Solid Edge part; units mm, degrees
sketch "Sketch1" plane through (0, 0, 0) normal (0, 0, 1) x (1, 0, 0)
  line L0 (0, 0) -> (50.8, 0)
  line L1 (50.8, 0) -> (50.8, 63.5)
  line L2 (50.8, 63.5) -> (0, 63.5)
  line L3 (0, 63.5) -> (0, 0)
extrude "Protrusion1" add sketch "Sketch1" along normal blind 3.175
hole "Hole_1" at (7.9375, 6.35, 0) direction (0, 0, 1) diameter 4.826 end up to next countersink diameter 9.525 countersink angle 82
hole "Hole1" at (42.8625, 6.35, 0) direction (0, 0, 1) diameter 4.826 end up to next countersink diameter 9.525 countersink angle 82
hole "Hole_2" at (25.4, 34.925, 3.175) direction (0, 0, -1) diameter 12.7 end up to next
chamfer "Chamfer_1" distance 6.35 angle 45 2 edges at (0, 63.5, 1.5875) (50.8, 63.5, 1.5875)
hole "Hole_4" at (14.4, 46.925, 0) direction (0, 0, 1) diameter 3.5 end up to next countersink diameter 6 countersink angle 90
hole "Hole2" at (14.4, 25.925, 0) direction (0, 0, 1) diameter 3.5 end up to next countersink diameter 6 countersink angle 90
hole "Hole3" at (36.4, 25.925, 0) direction (0, 0, 1) diameter 3.5 end up to next countersink diameter 6 countersink angle 90
hole "Hole4" at (36.4, 46.925, 0) direction (0, 0, 1) diameter 3.5 end up to next countersink diameter 6 countersink angle 90
properties part number "CHAS-04" material "Aluminum, 1060"
Work out the finished part from the listing and answer in its coordinate system (mm). Coordinates: 2 decimals unless noted, no trailing zeros. Write each loop counter-clockwise with the first axis right and the second up, starting at its lowest first coordinate (ties: lowest second). Pieces come first, ordered by that corner, then holes. Notation, with made-up numbers: (34, 70) - (57, 70) arc R20 ccw to (57, 84) - close; hole circle Ø7 at (62, 14). An arc over 180 degrees is marked (long way). One line per question, with ' | ' between items.
1) Find section A-A, the plane x = 14.4. Determine the outline of the cut face in (y, z) (3 decimals).
Checks:
outline: (0, 0) - (22.925, 0) - (24.175, 1.25) - (24.175, 3.175) - (0, 3.175) - close; (27.675, 1.25) - (28.925, 0) - (43.925, 0) - (45.175, 1.25) - (45.175, 3.175) - (27.675, 3.175) - close; (48.675, 1.25) - (49.925, 0) - (63.5, 0) - (63.5, 3.175) - (48.675, 3.175) - close
2) Find section B-B, the plane y = 6.35. Determine the outline of the cut face in (x, z) (1 decimal).
Checks:
outline: (0, 0) - (3.2, 0) - (5.5, 2.7) - (5.5, 3.2) - (0, 3.2) - close; (10.4, 2.7) - (12.7, 0) - (38.1, 0) - (40.4, 2.7) - (40.4, 3.2) - (10.4, 3.2) - close; (45.3, 2.7) - (47.6, 0) - (50.8, 0) - (50.8, 3.2) - (45.3, 3.2) - close
3) Find section C-C, the plane x = 25.4. Determine the outline of the cut face in (y, z) (3 decimals), and give its area (3 significant figures).
Checks:
outline: (0, 0) - (28.575, 0) - (28.575, 3.175) - (0, 3.175) - close; (41.275, 0) - (63.5, 0) - (63.5, 3.175) - (41.275, 3.175) - close | area: 161 mm2
4) The mould has two halves that part along Y. Classify faces 1 (the face through (25, 0, 2)), 2 (the face through (19, 32, 0)), 3 (the face through (41.882, 8.715, 2.534)), 4 (the face through (36.9, 27.6, 2.2)): +Y half, -Y half, draft (parallel to the pull), parting line (faces both ways), or undercut.
Checks:
face 1: -Y half | face 2: draft | face 3: undercut | face 4: undercut
5) Flat-ended cylindrical pins translate along their axes: P1, Ø4.5, axis at x = 14.4, y = 25.925, coming from the +Z side (3 decimals); P2, Ø1, axis at x = 40.5, y = 7.5, coming from the -Z side. Find the tip coordinate at first contact, or state that the pin passes through.
Checks:
P1: z = 3.175 | P2: z = 1.88
6) Find section D-D, the plane z = 1.9. Give the number of separate pieces and of enclosed holes in the cut face, and give its area (3 significant figures).
Checks:
separate pieces: 1 | enclosed holes: 7 | area: 2,960 mm2
7) Consider probe 1 along X at (y, z) = (6.35, 2.8); probe 2 along Y at (x, z) = (36.5, 2.2); probe 3 along Y at (x, z) = (25.4, 2) (3 decimals). Determine where each line is inside the solid, lowest interval first. Write a range as [from, to].
Checks:
probe 1: [0, 5.52], [10.35, 40.45], [45.28, 50.8] | probe 2: [0, 24.18], [27.67, 45.18], [48.67, 63.5] | probe 3: [0, 28.575], [41.275, 63.5]
